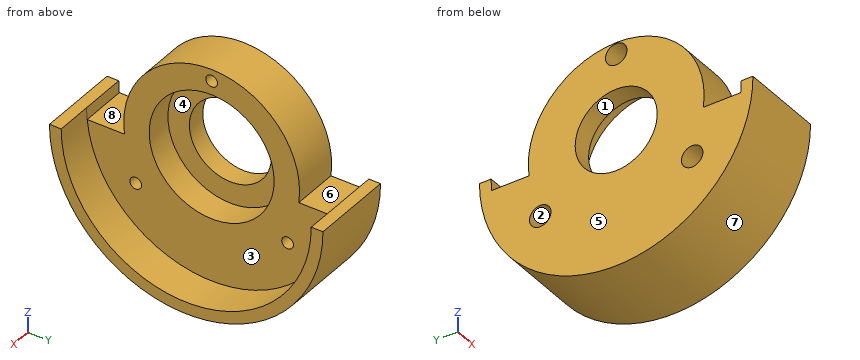
from build123d import *
from build123d.topology import SkipClean

# Parameters (mm, degrees)
CUT_EXTRUDE1_DEPTH      = 51.931326313
CUT_EXTRUDE1_DEPTH_BACK = 51.931326313
SKETCH2_R               = 1.5
SKETCH3_R               = 2.75
CUT_EXTRUDE2_DEPTH      = 5


with BuildPart() as part:
    # Sketch1 → Revolve1 (revolve)
    with BuildSketch(Plane.XY):
        Polygon((21.5, 35), (21.5, 32), (12, 32), (12, 16), (5, 16), (5, 10.5), (0, 10.5), (0, 35), align=None)
    revolve(axis=Axis((21.5, 0, 0), (-1, 0, 0)))

    # Sketch2 → Cut-Extrude1 (cut, two sides: drawn at the far end of the back side and taken through both)
    with SkipClean():  # the faces are left unmerged after this step: merging them gives an invalid solid
        with BuildSketch(Plane(origin=(12, 0, 0), x_dir=(0, 0, -1), z_dir=(1, 0, 0)).offset(-CUT_EXTRUDE1_DEPTH_BACK)):
            with Locations(Location((-19.5, 0, 0), (0, 0, 90))):
                Circle(SKETCH2_R)
            with Locations(Location((14.5, -19.437399517, 0), (0, 0, 90))):
                Circle(SKETCH2_R)
            with Locations(Location((14.5, 19.437399517, 0), (0, 0, 90))):
                Circle(SKETCH2_R)
            with BuildLine():
                Line((3, 22.299103121), (3, 31.859064644))
                ThreePointArc((3, 31.859064644), (1.501654319, 31.964746742), (0, 32))
                Line((0, 32), (0, 35))
                ThreePointArc((0, 35), (-35, 0), (0, -35))
                Line((0, -35), (0, -32))
                ThreePointArc((0, -32), (1.501654319, -31.964746742), (3, -31.859064644))
                Line((3, -31.859064644), (3, -22.299103121))
                ThreePointArc((3, -22.299103121), (-22.5, 0), (3, 22.299103121))
            make_face()
        extrude(amount=CUT_EXTRUDE1_DEPTH + CUT_EXTRUDE1_DEPTH_BACK, mode=Mode.SUBTRACT)

    # Sketch3 → Cut-Extrude2 (cut)
    with SkipClean():  # the faces are left unmerged after this step: merging them gives an invalid solid
        with BuildSketch(Plane.ZY):
            with Locations(Location((-14.5, 19.437399517, 0), (0, 0, 270))):
                Circle(SKETCH3_R)
            with Locations(Location((19.5, 0, 0), (0, 0, 270))):
                Circle(SKETCH3_R)
            with Locations(Location((-14.5, -19.437399517, 0), (0, 0, 270))):
                Circle(SKETCH3_R)
        extrude(amount=-CUT_EXTRUDE2_DEPTH, mode=Mode.SUBTRACT)


solid = part.part
For this review, take the finished solid that the model builds, in its own axes (mm). Face numbers are marked on the shaded views. A direction names the side the tool comes from. Coordinates: 2 decimals unless noted, no trailing zeros. Loops run counter-clockwise (first coordinate to the right, second up) from the corner with the lowest first, then second, coordinate; pieces in that order, holes last. Notation, with made-up numbers: (38, 49) - (48, 49) arc R21 ccw to (48, 83) - close; hole circle Ø11 at (69, 10.25). An arc over 180 degrees is marked (long way). Use a Markdown table: item, result. Add a question column.
Item 1: Insertion check: pin 1 Ø3 at (y, z) = (0, 20.5) entering from -X; pin 2 Ø3.5 at (x, y) = (13, -34) entering from +Z; pin 3 Ø5 at (x, y) = (17, -5.5) entering from -Z. Each pin has a flat end and moves straight along its axis. Give the tip position at first contact, or say it passes through.
Item 2: We need section A-A (y = 0). Give the boundary of the cut face in (x, z), and give its area (3 significant figures).
Item 3: Tool access review of the marked faces 1, 2, 3 and 4: name each direction out of +Z, -Z, +X, -X, +Y, -Y from which nothing blocks a thin tool from reaching the whole face with its end or side.
Item 4: For line 1 (X direction, y = 9, z = -30.5); line 2 (X direction, y = -11, z = 4); line 3 (Y direction, x = 8.5, z = -14.5), list the stretches that pass through material, from the lowest coordinate up.
Item 5: We need section B-B (x = 7). Give the boundary of the cut face in (y, z), and give its area (3 significant figures).
Item 6: Mouldability with a two-part tool opening along Y and no side actions: class the marked faces 5, 6, 7 and 8 as pulls with the +Y half, pulls with the -Y half, needs draft (parallel to the pull), parting line crosses it, or undercut.
Item 7: We need section D-D (y = 20). Give the boundary of the cut face in (x, z), and give its area (3 significant figures).
Item 8: We need section C-C (z = -14.5). Give the boundary of the cut face in (x, y), and give its area (3 significant figures).
Results list:
| question | item | result |
|---|---|---|
| 1 | pin 1 | stops at x = 5 |
| 1 | pin 2 | stops at z = 0 |
| 1 | pin 3 | stops at z = -34.87 |
| 2 | outline | (0, -35) - (21.5, -35) - (21.5, -32) - (12, -32) - (12, -16) - (5, -16) - (5, -10.5) - (0, -10.5) - close; (0, 10.5) - (5, 10.5) - (5, 16) - (12, 16) - (12, 18) - (5, 18) - (5, 16.75) - (0, 16.75) - close; (0, 22.25) - (5, 22.25) - (5, 21) - (12, 21) - (12, 22.5) - (0, 22.5) - close |
| 2 | area | 341 mm^2 |
| 3 | face 1 | +X, -X |
| 3 | face 2 | -X |
| 3 | face 3 | +Z, +X |
| 3 | face 4 | +X |
| 4 | line 1 | x = 0 to 12 |
| 4 | line 2 | x = 0 to 5 |
| 4 | line 3 | y = -31.86 to -20.94, -17.94 to -6.76, 6.76 to 17.94, 20.94 to 31.86 |
| 5 | outline | (-35, 0) arc R35 ccw to (35, 0) - (32, 0) arc R32 cw to (31.86, -3) - (22.3, -3) arc R22.5 ccw (long way) to (-22.3, -3) - (-31.86, -3) arc R32 cw to (-32, 0) - close; hole circle Ø3 at (-19.44, -14.5); hole circle Ø32 at (0, 0); hole circle Ø3 at (0, 19.5); hole circle Ø3 at (19.44, -14.5) |
| 5 | area | 1,840 mm^2 |
| 6 | face 5 | needs draft |
| 6 | face 6 | undercut |
| 6 | face 7 | parting line crosses it |
| 6 | face 8 | undercut |
| 7 | outline | (0, -28.72) - (21.5, -28.72) - (21.5, -24.98) - (12, -24.98) - (12, -15.89) - (5, -15.89) - (5, -17.19) - (0, -17.19) - close; (0, -11.81) - (5, -11.81) - (5, -13.11) - (12, -13.11) - (12, 10.31) - (0, 10.31) - close |
| 7 | area | 458 mm^2 |
| 8 | outline | (0, -31.86) - (21.5, -31.86) - (21.5, -28.53) - (12, -28.53) - (12, -20.94) - (5, -20.94) - (5, -22.19) - (0, -22.19) - close; (0, -16.69) - (5, -16.69) - (5, -17.94) - (12, -17.94) - (12, -6.76) - (5, -6.76) - (5, 6.76) - (12, 6.76) - (12, 17.94) - (5, 17.94) - (5, 16.69) - (0, 16.69) - close; (0, 22.19) - (5, 22.19) - (5, 20.94) - (12, 20.94) - (12, 28.53) - (21.5, 28.53) - (21.5, 31.86) - (0, 31.86) - close |
| 8 | area | 636 mm^2 |
